Work out the finished part from the listing and answer in its coordinate system (mm). A direction names the side the tool comes from. Round coordinates to 2 decimals unless told otherwise and drop trailing zeros. Order: outer loops, then holes, each group sorted by start corner. A loop starts at its lowest first (then second) coordinate and runs counter-clockwise, first axis right, second up. Notation, with made-up numbers: (-30, -27) - (-7, -27) arc R16 cw to (-7, -23) - close; hole circle Ø1 at (-3.5, -11). An arc over 180 degrees is marked (long way). Answer in a Markdown table with one row per item.
from build123d import *

# Parameters (mm, degrees)
ESQUISSE1_W                = 130
ESQUISSE1_H                = 50
BOSS_EXTRU_1_DEPTH         = 3.175
ESQUISSE2_W                = 3.175
ESQUISSE2_H                = 10
BOSS_EXTRU_2_DEPTH         = 3.175
ESQUISSE3_W                = 20
ESQUISSE3_H                = 3.175
ENL_V_MAT_EXTRU_1_DEPTH    = 3.175
ESQUISSE4_W                = 10
ESQUISSE4_H                = 3.175
BOSS_EXTRU_3_DEPTH         = 3.175
R_P_TITION_LIN_AIRE1_COUNT = 7
R_P_TITION_LIN_AIRE1_PITCH = 20


with BuildPart() as part:
    # Esquisse1 → Boss.-Extru.1 (new body)
    with BuildSketch(Plane.XY):
        with Locations((65, 25)):
            Rectangle(ESQUISSE1_W, ESQUISSE1_H)
    extrude(amount=BOSS_EXTRU_1_DEPTH)

    # Esquisse2 → Boss.-Extru.2 (add)
    with BuildSketch(Plane.XY.offset(3.175)):
        with Locations((131.5875, 35)):
            Rectangle(ESQUISSE2_W, ESQUISSE2_H)
        with Locations((131.5875, 15)):
            Rectangle(ESQUISSE2_W, ESQUISSE2_H)
        with Locations((-1.5875, 35)):
            Rectangle(ESQUISSE2_W, ESQUISSE2_H)
        with Locations((-1.5875, 15)):
            Rectangle(ESQUISSE2_W, ESQUISSE2_H)
    extrude(amount=-BOSS_EXTRU_2_DEPTH)

    # Esquisse3 → Enlèv. mat.-Extru.1 (cut)
    with BuildSketch(Plane.XY.offset(3.175)):
        with Locations((65, 48.4125)):
            Rectangle(ESQUISSE3_W, ESQUISSE3_H)
    extrude(amount=-ENL_V_MAT_EXTRU_1_DEPTH, mode=Mode.SUBTRACT)

    # Esquisse4 → Boss.-Extru.3 (add)
    with BuildSketch(Plane.XY.offset(3.175)):
        with Locations((5, -1.5875)):
            Rectangle(ESQUISSE4_W, ESQUISSE4_H)
    boss_extru_3 = extrude(amount=-BOSS_EXTRU_3_DEPTH)

    # Répétition linéaire1: Boss.-Extru.3 ×7
    with Locations(*[(i * R_P_TITION_LIN_AIRE1_PITCH, 0, 0) for i in range(1, R_P_TITION_LIN_AIRE1_COUNT)]):
        add(boss_extru_3)


solid = part.part
1) Which of the six approach directions +Z, -Z, +X, -X, +Y, -Y give full straight-line access (tool end or side, diameter ignored) to faces 1 (the face through (130, 45, 2)), 2 (the face through (110, -2, 2)), 3 (the face through (-2, 40, 2)), 4 (the face through (-2, 30, 2))?
Filled in:
| item | result |
|---|---|
| face 1 | +Z, -Z, +X, +Y |
| face 2 | +Z, -Z, -Y |
| face 3 | +Z, -Z, -X, +Y |
| face 4 | +Z, -Z, -X |
2) Find section B-B, the plane x = 15.5. Give the vertices of the cut face in (y, z) (3 decimals), then the cut area to 3 significant figures.
Filled in:
| item | result |
|---|---|
| outline | (0, 0) - (50, 0) - (50, 3.175) - (0, 3.175) - close |
| area | 159 mm^2 |
3) Find section A-A, the plane y = 21.5. Give the vertices of the cut face in (x, z) (3 decimals), then the cut area to 3 significant figures.
Filled in:
| item | result |
|---|---|
| outline | (0, 0) - (130, 0) - (130, 3.175) - (0, 3.175) - close |
| area | 413 mm^2 |
4) Find the intervals of material crossed by probe 1 along X at (y, z) = (4.5, 1.85); probe 2 along Y at (x, z) = (117, 0.3); probe 3 along Y at (x, z) = (67.5, 2.75) (3 decimals), in increasing order. Write a range as from..to.
Filled in:
| item | result |
|---|---|
| probe 1 | x = 0..130 |
| probe 2 | y = 0..50 |
| probe 3 | y = -3.175..46.825 |
5) Each of these flat-tipped pins is pushed along its axis until it touches: pin 1 (1 mm diameter, centred on x = 131, z = 2, fed in from +Y); pin 2 (1.6 mm diameter, centred on y = 48.5, z = 1.5, fed in from -X); pin 3 (1.5 mm diameter, centred on x = 95, z = 1, fed in from -Y). Where does it stop, or does it pass through?
Filled in:
| item | result |
|---|---|
| pin 1 | stops at y = 40 |
| pin 2 | stops at x = 0 |
| pin 3 | stops at y = 0 |
